Autodesk Fusion 360 part; units mm, degrees
sketch "Sketch1" plane through (0, 0, 0) normal (0, 0, 1) x (1, 0, 0)
  line L0 (0, 0) -> (-60, 0)
  line L1 (-60, 0) -> (60, 0)
  line L2 (-60, 0) -> (-60, 40)
  line L3 (60, 0) -> (60, -40)
  line L4 (-60, 40) -> (60, 40)
  line L5 (60, 40) -> (60, -40)
  line L6 (60, -40) -> (-60, -40)
  line L7 (-60, -40) -> (-60, 40)
  dimension "d1" = 60
  dimension "d2" = 120
  dimension "d3" = 40
  dimension "d4" = 40
extrude "Extrude1" add sketch "Sketch1" along normal blind 35
sketch "Sketch2" plane through (0, 0, 35) normal (0, 0, 1) x (-1, 0, 0)
  line L0 (60, 40) -> (-60, 40)
  line L1 (-60, 40) -> (-60, -40)
  line L2 (-60, -40) -> (60, -40)
  line L3 (60, -40) -> (60, 40)
  line L4 (-60, -40) -> (40, -40)
  line L5 (60, 0) -> (60, -15)
  line L6 (60, 0) -> (60, 15)
  circle A0 centre (40, -15) radius 8.5
  circle A1 centre (40, 15) radius 8.5
  dimension "d10" = 17
  dimension "d11" = 17
extrude "Extrude2" cut sketch "Sketch2" against normal blind 70 contours A0 | A1
sketch "Sketch3" plane through (0, 0, 35) normal (0, 0, 1) x (-1, 0, 0)
  circle A0 centre (40, -15) radius 8.5
  circle A1 centre (40, 15) radius 8.5
  line L0 (60, 40) -> (-60, 40)
  line L1 (-60, 40) -> (-60, -40)
  line L2 (-60, -40) -> (60, -40)
  line L3 (60, -40) -> (60, 40)
  line L4 (-60, 40) -> (0, 40)
  circle A2 centre (0, 0) radius 9
  dimension "d14" = 60
  dimension "d15" = 18
extrude "Extrude3" cut sketch "Sketch3" against normal blind 55 contours A2
sketch "Sketch4" plane through (0, 0, 35) normal (0, 0, 1) x (-1, 0, 0)
  circle A0 centre (0, 0) radius 9
  circle A1 centre (40, -15) radius 8.5
  circle A2 centre (40, 15) radius 8.5
  line L0 (60, 40) -> (-60, 40)
  line L1 (-60, 40) -> (-60, -40)
  line L2 (-60, -40) -> (60, -40)
  line L3 (60, -40) -> (60, 40)
  circle A3 centre (0, 0) radius 15
  dimension "d18" = 30
extrude "Extrude4" cut sketch "Sketch4" against normal blind 17 contours A3
sketch "Sketch5" plane through (0, 40, 0) normal (0, 1, 0) x (-1, 0, 0)
  line L0 (-60, 0) -> (60, 0)
  line L1 (60, 0) -> (60, 35)
  line L2 (60, 35) -> (-60, 35)
  line L3 (-60, 35) -> (-60, 0)
  line L4 (-60, 0) -> (-40, 0)
  line L5 (-60, 0) -> (-60, 50)
  line L6 (-20, 50) -> (-20, 0)
  arc A0 (-20, 50) -> (-60, 50) centre (-40, 50) ccw
  dimension "d21" = 20
  dimension "d22" = 50
  dimension "d23" = 40
extrude "Extrude5" add sketch "Sketch5" against normal blind 80 contours L0 L2 L3 L4 L5 L6 | L2 L5 L6 A0
sketch "Sketch6" plane through (0, 40, 0) normal (0, 1, 0) x (-1, 0, 0)
  line L0 (-60, 0) -> (60, 0)
  line L1 (60, 0) -> (60, 35)
  line L2 (60, 35) -> (-20, 35)
  line L3 (-20, 35) -> (-20, 50)
  arc A0 (-20, 50) -> (-60, 50) centre (-40, 50) ccw
  line L4 (-60, 50) -> (-60, 0)
  circle A1 centre (-40, 50) radius 10
  dimension "d26" = 20
extrude "Extrude6" cut sketch "Sketch6" against normal blind 95 contours A1
sketch "Sketch7" plane through (0, 0, 35) normal (0, 0, 1) x (-1, 0, 0)
  line L0 (-20, 40) -> (-20, -40)
  line L1 (-20, -40) -> (60, -40)
  line L2 (60, -40) -> (60, 40)
  line L3 (60, 40) -> (-20, 40)
  circle A0 centre (0, 0) radius 15
  circle A1 centre (40, -15) radius 8.5
  circle A2 centre (40, 15) radius 8.5
  line L4 (60, 40) -> (60, 30) construction
  line L5 (60, -40) -> (60, -30) construction
  line L6 (60, -40) -> (-20, -40)
  line L7 (-20, -40) -> (-20, -30)
  line L8 (-20, -30) -> (60, -30)
  line L9 (60, -30) -> (60, -40)
  line L10 (60, 30) -> (-20, 30)
  line L11 (-20, 30) -> (-20, 40)
  line L12 (-20, 40) -> (60, 40)
  line L13 (60, 40) -> (60, 30)
extrude "Extrude7" cut sketch "Sketch7" against normal blind 5 contours L0 L2 L3 L10 L11 L12 L13 | L0 L1 L2 L6 L7 L8 L9
ref_plane "WorkPlane1" through (0, 0, 35) normal (0, 0, 1) x (1, 0, 0)
sketch "Sketch8" plane through (0, 0, 35) normal (0, 0, 1) x (1, 0, 0)
  line L0 (60, -40) -> (-60, -40)
  line L1 (-60, -40) -> (-60, 40)
  line L2 (-60, 40) -> (60, 40)
  line L3 (60, 40) -> (60, -40)
  circle A0 centre (-40, -15) radius 8.5
  circle A1 centre (-40, 15) radius 8.5
  circle A2 centre (0, 0) radius 9
  line L4 (60, 0) -> (30, 0) construction
  line L5 (30, 0) -> (20, 0) construction
  line L6 (20, 0) -> (20, 10) construction
  line L7 (20, 10) -> (20, -10)
  line L8 (20, -10) -> (67.6256, -10)
  line L9 (67.6256, -10) -> (67.6256, 10)
  line L10 (67.6256, 10) -> (20, 10)
  dimension "d33" = 30
  dimension "d34" = 10
  dimension "d35" = 20
extrude "Extrude8" cut sketch "Sketch8" along normal blind 90 contours L3 L7 L8 L10 | L3 L8 L9 L10
sketch "Sketch9" plane through (0, 0, 0) normal (0, 0, -1) x (1, 0, 0)
  line L0 (60, 40) -> (-60, 40)
  line L1 (-60, 40) -> (-60, -40)
  line L2 (-60, -40) -> (60, -40)
  line L3 (60, -40) -> (60, 40)
  circle A0 centre (-40, 15) radius 8.5
  circle A1 centre (-40, -15) radius 8.5
  circle A2 centre (0, 0) radius 9
  line L4 (60, 0) -> (20, 0) construction
  line L5 (60, 0) -> (30, 0) construction
  line L6 (30, -10) -> (73.1497, -10)
  arc A3 (73.1497, -10) -> (73.1497, 10) centre (73.1497, 0) ccw
  line L7 (73.1497, 10) -> (30, 10)
  arc A4 (30, 10) -> (30, -10) centre (30, 0) ccw
  line L8 (20, 0) -> (83.1497, 0) construction
  dimension "d38" = 40
  dimension "d39" = 30
  dimension "d40" = 20
extrude "Extrude9" cut sketch "Sketch9" against normal blind 13 contours L3 L6 L7 A4
Read the model definition and answer for the solid it produces. Units are mm, in the model's axes. A direction names the side the tool comes from. Coordinates: 2 decimals unless noted, no trailing zeros. Loops run counter-clockwise (first coordinate to the right, second up) from the corner with the lowest first, then second, coordinate; pieces in that order, holes last. Notation, with made-up numbers: (-2, -10.75) -> (3, -10.75) arc R29 ccw to (3, 13.25) -> close; hole circle Ø8 at (31.25, 0). An arc over 180 degrees is marked (long way). Answer in a Markdown table with one row per item.
Item 1: For faces 4 (the flat face through (-19, 35, 30)), 5 (the flat face through (45, 10, 6)), 6 (the cylindrical face through (14.985, -0.66, 26.619)), 7 (the flat face through (44, -10, 60)), determine the directions among +Z, -Z, +X, -X, +Y, -Y from which every point of the face is accessible in a straight line to the end or side of a thin tool.
Returned:
| item | result |
|---|---|
| face 4 | +Z, -X, +Y |
| face 5 | -Z, +X |
| face 6 | +Z |
| face 7 | +Z, +X, -X |
Item 2: Each of these flat-tipped pins is pushed along its axis until it touches: P1, Ø10, axis at y = -24.5, z = 57.5, coming from the -X side; P2, Ø2.5, axis at x = -23, z = 31.5, coming from the +Y side; P3, Ø8, axis at x = -10, y = 32.5, coming from the +Z side. Where does it stop, or does it pass through?
Returned:
| item | result |
|---|---|
| P1 | stops at x = 20.16 |
| P2 | stops at y = 30 |
| P3 | stops at z = 35 |
Item 3: For a pull along X with two mould halves and no side action, classify faces 1 (the cylindrical face through (20, 0, 6)), 2 (the flat face through (40, 0, 13)), 3 (the flat face through (-6.5, 6.5, 18)) as released by +X, released by -X, zero draft, split by the parting line, or undercut.
Returned:
| item | result |
|---|---|
| face 1 | released by +X |
| face 2 | zero draft |
| face 3 | undercut |
Item 4: A cutting plane is placed at A-A on x = 0. Determine the outline of the cut face in (y, z).
Returned:
| item | result |
|---|---|
| outline | (-40, 0) -> (-9, 0) -> (-9, 18) -> (-15, 18) -> (-15, 35) -> (-30, 35) -> (-30, 30) -> (-40, 30) -> close; (9, 0) -> (40, 0) -> (40, 30) -> (30, 30) -> (30, 35) -> (15, 35) -> (15, 18) -> (9, 18) -> close |
Item 5: Straight lines are drawn through the part: line 1 along Y through (x, z) = (-40, 12); line 2 along Y through (x, z) = (0, 25.75); line 3 along X through (y, z) = (-15, 15.5). For each, find the intervals that lie inside material, in ascending order. Write a range as [from, to].
Returned:
| item | result |
|---|---|
| line 1 | y = [-40, -23.5], [-6.5, 6.5], [23.5, 40] |
| line 2 | y = [-40, -15], [15, 40] |
| line 3 | x = [-60, -48.5], [-31.5, 60] |
Item 6: A cutting plane is placed at D-D on z = 5.5. Determine the outline of the cut face in (x, y), plus the area to 3 significant figures.
Returned:
| item | result |
|---|---|
| outline | (-60, -40) -> (60, -40) -> (60, -10) -> (30, -10) arc R10 cw to (30, 10) -> (60, 10) -> (60, 40) -> (-60, 40) -> close; hole circle Ø17 at (-40, -15); hole circle Ø17 at (-40, 15); hole circle Ø18 at (0, 0) |
| area | 8,130 mm^2 |
Item 7: A cutting plane is placed at C-C on x = 40. Determine the outline of the cut face in (y, z), plus the area to 3 significant figures.
Returned:
| item | result |
|---|---|
| outline | (-40, 0) -> (-10, 0) -> (-10, 13) -> (10, 13) -> (10, 0) -> (40, 0) -> (40, 40) -> (10, 40) -> (10, 35) -> (-10, 35) -> (-10, 40) -> (-40, 40) -> close; (-40, 60) -> (-10, 60) -> (-10, 70) -> (-40, 70) -> close; (10, 60) -> (40, 60) -> (40, 70) -> (10, 70) -> close |
| area | 3,440 mm^2 |
Item 8: A cutting plane is placed at B-B on y = 0. Determine the outline of the cut face in (x, z).
Returned:
| item | result |
|---|---|
| outline | (-60, 0) -> (-9, 0) -> (-9, 18) -> (-15, 18) -> (-15, 35) -> (-60, 35) -> close; (9, 0) -> (20, 0) -> (20, 13) -> (60, 13) -> (60, 35) -> (15, 35) -> (15, 18) -> (9, 18) -> close |
